Work out the finished part from the listing and answer in its coordinate system (mm). Face numbers are marked on the shaded views. Coordinates: 2 decimals unless noted, no trailing zeros. Loops run counter-clockwise (first coordinate to the right, second up) from the corner with the lowest first, then second, coordinate; pieces in that order, holes last. Notation, with made-up numbers: (63, -12.5) -> (116, -12.5) arc R8 ccw to (116, -1.5) -> close; hole circle Ø5 at (82, -13.75). An arc over 180 degrees is marked (long way). Use a Markdown table: item, result.
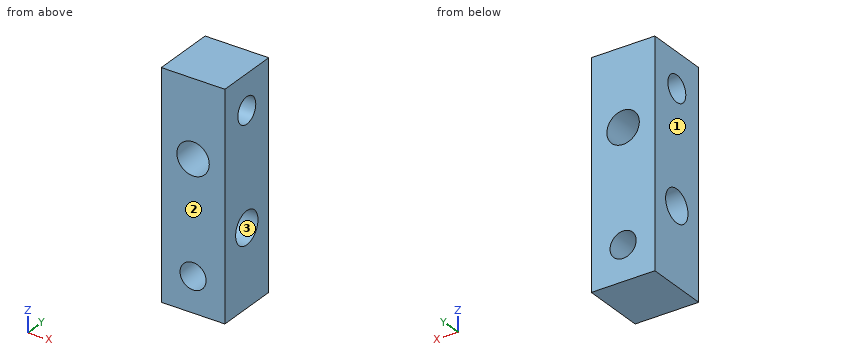
from build123d import *

# Parameters (mm, degrees)
F0_W     = 20
F0_H     = 20
F1_DEPTH = 70
F2_R     = 5.1
F2_R_2   = 4.1
F3_DEPTH = 20.001
F4_R     = 5.1
F4_R_2   = 4.1
F5_DEPTH = 20.001


with BuildPart() as f1:
    # F0 (on Top) → F1 (new body)
    with BuildSketch(Plane.XY):
        Rectangle(F0_W, F0_H)
    extrude(amount=F1_DEPTH)

    # F2 (on face) → F3 (cut, through all)
    with BuildSketch(Plane.XZ.offset(10)):
        with Locations((0, 46)):
            Circle(F2_R)
        with Locations((0, 11)):
            Circle(F2_R_2)
    extrude(amount=-F3_DEPTH, mode=Mode.SUBTRACT)

    # F4 (on face) → F5 (cut, through all)
    with BuildSketch(Plane.YZ.offset(10)):
        with Locations((0, 24)):
            Circle(F4_R)
        with Locations((0, 59)):
            Circle(F4_R_2)
    extrude(amount=-F5_DEPTH, mode=Mode.SUBTRACT)


solid = f1.part
Q1. Consider line 1 (Z direction, x = 5.75, y = 0); line 2 (Z direction, x = -0.5, y = 5.25); line 3 (Z direction, x = 0, y = -1.75). Determine where each line is inside the solid, lowest interval first. Write a range as [from, to].
Solved:
| item | result |
|---|---|
| line 1 | [0, 18.9], [29.1, 54.9], [63.1, 70] |
| line 2 | [0, 6.93], [15.07, 40.92], [51.08, 70] |
| line 3 | [0, 6.9], [15.1, 19.21], [28.79, 40.9], [51.1, 55.29], [62.71, 70] |
Q2. Section D-D on y = 6 is taken. Determine the outline of the cut face in (x, z).
Solved:
| item | result |
|---|---|
| outline | (-10, 0) -> (10, 0) -> (10, 70) -> (-10, 70) -> close; hole circle Ø10.2 at (0, 46); hole circle Ø8.2 at (0, 11) |
Q3. Section C-C on z = 46 is taken. Determine the outline of the cut face in (x, y), and give its area (3 significant figures).
Solved:
| item | result |
|---|---|
| outline | (-10, -10) -> (-5.1, -10) -> (-5.1, 10) -> (-10, 10) -> close; (5.1, -10) -> (10, -10) -> (10, 10) -> (5.1, 10) -> close |
| area | 196 mm² |
Q4. Section B-B on y = 0 is taken. Determine the outline of the cut face in (x, z).
Solved:
| item | result |
|---|---|
| outline | (-10, 0) -> (10, 0) -> (10, 18.9) -> (-10, 18.9) -> close; (-10, 29.1) -> (10, 29.1) -> (10, 54.9) -> (-10, 54.9) -> close; (-10, 63.1) -> (10, 63.1) -> (10, 70) -> (-10, 70) -> close; hole circle Ø10.2 at (0, 46); hole circle Ø8.2 at (0, 11) |
Q5. Section A-A on x = 0 is taken. Determine the outline of the cut face in (y, z).
Solved:
| item | result |
|---|---|
| outline | (-10, 0) -> (10, 0) -> (10, 6.9) -> (-10, 6.9) -> close; (-10, 15.1) -> (10, 15.1) -> (10, 40.9) -> (-10, 40.9) -> close; (-10, 51.1) -> (10, 51.1) -> (10, 70) -> (-10, 70) -> close; hole circle Ø10.2 at (0, 24); hole circle Ø8.2 at (0, 59) |
Q6. Determine the mould class of the marked faces 1, 2 and 3 for opening direction Y: pulls with the +Y half, pulls with the -Y half, needs draft (parallel to the pull), parting line crosses it, or undercut.
Solved:
| item | result |
|---|---|
| face 1 | needs draft |
| face 2 | pulls with the -Y half |
| face 3 | undercut |
